from build123d import *

# Parameters (mm, degrees)
SKETCH1_W           = 48
SKETCH1_H           = 25
SKETCH1_W_2         = 5
SKETCH1_H_2         = 1.5
SKETCH1_H_3         = 5
BOSS_EXTRUDE1_DEPTH = 1.6
SKETCH3_R           = 1
BOSS_EXTRUDE2_DEPTH = 0.5
SKETCH4_R           = 0.75
BOSS_EXTRUDE3_DEPTH = 4.5
SKETCH5_R           = 0.45
BOSS_EXTRUDE4_DEPTH = 2
FILLET1_R           = 0.45
SKETCH6_W           = 3
SKETCH6_H           = 25
CUT_EXTRUDE1_DEPTH  = 10


with BuildPart() as part:
    # Sketch1 → Boss-Extrude1 (new body)
    with BuildSketch(Plane(origin=(0, 0, 0), x_dir=(1, 0, 0), z_dir=(0, 1, 0))):
        Rectangle(SKETCH1_W, SKETCH1_H)
        with Locations((15.5, 3.5)):
            Rectangle(SKETCH1_W_2, SKETCH1_H_2, mode=Mode.SUBTRACT)
        with Locations((15.5, -1.25)):
            Rectangle(SKETCH1_W_2, SKETCH1_H_3, mode=Mode.SUBTRACT)
        with Locations((-15.5, 9.5)):
            Rectangle(SKETCH1_W_2, SKETCH1_H_2, mode=Mode.SUBTRACT)
        with Locations((15.5, 9.5)):
            Rectangle(SKETCH1_W_2, SKETCH1_H_2, mode=Mode.SUBTRACT)
        with Locations((15.5, 6.5)):
            Rectangle(SKETCH1_W_2, SKETCH1_H_2, mode=Mode.SUBTRACT)
        with Locations((15.5, -7.75)):
            Rectangle(SKETCH1_W_2, SKETCH1_H_3, mode=Mode.SUBTRACT)
        with Locations((-15.5, -7.75)):
            Rectangle(SKETCH1_W_2, SKETCH1_H_3, mode=Mode.SUBTRACT)
        with Locations((-15.5, 6.5)):
            Rectangle(SKETCH1_W_2, SKETCH1_H_2, mode=Mode.SUBTRACT)
    extrude(amount=BOSS_EXTRUDE1_DEPTH)

    # Sketch3 → Boss-Extrude2 (add)
    with BuildSketch(Plane.XZ):
        with Locations(Location((0, 0, 0), (0, 0, 90))):
            Circle(SKETCH3_R)
        with Locations(Location((0, -5, 0), (0, 0, 90))):
            Circle(SKETCH3_R)
    extrude(amount=BOSS_EXTRUDE2_DEPTH)

    # Sketch4 → Boss-Extrude3 (add)
    with BuildSketch(Plane.XZ.offset(0.5)):
        with Locations(Location((0, 0, 0), (0, 0, 270))):
            Circle(SKETCH4_R)
        with Locations(Location((0, -5, 0), (0, 0, 270))):
            Circle(SKETCH4_R)
    extrude(amount=BOSS_EXTRUDE3_DEPTH)

    # Sketch5 → Boss-Extrude4 (add)
    with BuildSketch(Plane.XZ.offset(5)):
        with Locations(Location((0, 0, 0), (0, 0, 270))):
            Circle(SKETCH5_R)
        with Locations(Location((0, -5, 0), (0, 0, 270))):
            Circle(SKETCH5_R)
    extrude(amount=BOSS_EXTRUDE4_DEPTH)

    # Fillet1
    fillet1_edges = [part.edges().sort_by_distance(p)[0] for p in [
        (0, -7, 0.45),
        (0, -7, -4.55),
    ]]
    fillet(fillet1_edges, radius=FILLET1_R)

    # Sketch6 → Cut-Extrude1 (cut)
    with BuildSketch(Plane.XZ):
        with Locations((-22.5, 0)):
            Rectangle(SKETCH6_W, SKETCH6_H)
        with Locations((22.5, 0)):
            Rectangle(SKETCH6_W, SKETCH6_H)
    extrude(amount=-CUT_EXTRUDE1_DEPTH, mode=Mode.SUBTRACT)


solid = part.part
Model file for the job. Use its own axes, mm. A direction names the side the tool comes from. Give positions to 0.01 mm unless a question says otherwise; leave off trailing zeros. Loops run counter-clockwise (first coordinate to the right, second up) from the corner with the lowest first, then second, coordinate; pieces in that order, holes last.
1) Pull direction Z, two halves, no side cores. Call faces 1 (the flat face through (-21, 1, 0)), 2 (the flat face through (15, 1, -7.25)), 3 (the flat face through (0, 1, -12.5)): +Z half, -Z half, draft (parallel to the pull), parting line (faces both ways), or undercut.
2) Saw through at A-A (x = 16). Write the cut outline in (y, z).
3) Tool access for faces 4 (the cylindrical face through (-0.172, -5.764, -0.416)), 5 (the flat face through (-18, 1, 8)): list every direction of +Z, -Z, +X, -X, +Y, -Y with a clear straight run to the whole face (end or side of a thin tool).
4) Wall check: line 1 (Y direction, x = -9.5, z = 0.75); line 2 (Z direction, x = -0.5, y = -4.5); line 3 (X direction, y = -4.75, z = 0). Give the ranges that are in metal, low to high.
5) Flat gauge pins, fed straight in: pin 1 Ø3 at (x, y) = (-13, -0.5) entering from -Z; pin 2 Ø5 at (y, z) = (-5, -2) entering from +X; pin 3 Ø1.5 at (x, z) = (-15.5, -5.5) entering from -Y. Where does each tip first touch, or does it go through?
6) Saw through at B-B (z = 2.75). Write the cut outline in (x, y).
7) Saw through at D-D (x = 0). Write the cut outline in (y, z), plus the area to 3 significant figures.
8) Saw through at C-C (z = -9.25). Write the cut outline in (x, y), plus the area to 3 significant figures.
Answer block:
1. face 1: draft
1. face 2: undercut
1. face 3: -Z half
2. outline: (0, -12.5) - (1.6, -12.5) - (1.6, -10.25) - (0, -10.25) - close; (0, -8.75) - (1.6, -8.75) - (1.6, -7.25) - (0, -7.25) - close; (0, -5.75) - (1.6, -5.75) - (1.6, -4.25) - (0, -4.25) - close; (0, -2.75) - (1.6, -2.75) - (1.6, -1.25) - (0, -1.25) - close; (0, 3.75) - (1.6, 3.75) - (1.6, 5.25) - (0, 5.25) - close; (0, 10.25) - (1.6, 10.25) - (1.6, 12.5) - (0, 12.5) - close
3. face 4: -Y
3. face 5: +Y, -Y
4. line 1: y = 0 to 1.6
4. line 2: z = -5.56 to -4.44, -0.56 to 0.56
4. line 3: x = -0.75 to 0.75
5. pin 1: stops at z = -12.5
5. pin 2: stops at x = 0.75
5. pin 3: stops at y = 0
6. outline: (-21, 0) - (13, 0) - (13, 1.6) - (-21, 1.6) - close; (18, 0) - (21, 0) - (21, 1.6) - (18, 1.6) - close
7. outline: (-6.55, -5.45) - (-5, -5.45) - (-5, -5.75) - (-0.5, -5.75) - (-0.5, -6) - (0, -6) - (0, -12.5) - (1.6, -12.5) - (1.6, 12.5) - (0, 12.5) - (0, 1) - (-0.5, 1) - (-0.5, 0.75) - (-5, 0.75) - (-5, 0.45) - (-6.55, 0.45) arc R0.45 ccw to (-6.55, -0.45) - (-5, -0.45) - (-5, -0.75) - (-0.5, -0.75) - (-0.5, -1) - (0, -1) - (0, -4) - (-0.5, -4) - (-0.5, -4.25) - (-5, -4.25) - (-5, -4.55) - (-6.55, -4.55) arc R0.45 ccw to start
7. area: 58.9 mm2
8. outline: (-21, 0) - (-18, 0) - (-18, 1.6) - (-21, 1.6) - close; (-13, 0) - (13, 0) - (13, 1.6) - (-13, 1.6) - close; (18, 0) - (21, 0) - (21, 1.6) - (18, 1.6) - close
8. area: 51.2 mm2
